Check sheet for the modelled part. Datum: model origin and axes. Units: mm. Face numbers are marked on the shaded views. A direction names the side the tool comes from. Coordinates: 2 decimals unless noted, no trailing zeros. Loops run counter-clockwise (first coordinate to the right, second up) from the corner with the lowest first, then second, coordinate; pieces in that order, holes last. Notation, with made-up numbers: (50.5, 59.25) -> (86.5, 59.25) arc R20 ccw to (86.5, 76.25) -> close; hole circle Ø3 at (82, -35.5). An arc over 180 degrees is marked (long way). Use one line per item in the form item = value.
from build123d import *

# Parameters (mm, degrees)
SKETCH1_R                       = 19.8
BOSS_EXTRUDE1_DEPTH             = 92
M4X0_7_TAPPED_HOLE1_D           = 3.3
M4X0_7_TAPPED_HOLE1_DEPTH       = 4
M4X0_7_TAPPED_HOLE1_CSINK_D     = 4.05
M4X0_7_TAPPED_HOLE1_CSINK_ANGLE = 90
M4X0_7_TAPPED_HOLE1_TIP         = 0.991420021
SKETCH6_R                       = 4
BOSS_EXTRUDE2_DEPTH             = 24
CHAMFER1_SIZE                   = 3
SKETCH7_W                       = 3.175
SKETCH7_H                       = 3.175
CUT_EXTRUDE1_DEPTH              = 19
CUT_EXTRUDE2_START              = -0.9
SKETCH8_R                       = 4
SKETCH8_R_2                     = 3.8
CUT_EXTRUDE2_DEPTH              = 0.9


with BuildPart() as part:
    # Sketch1 → Boss-Extrude1 (new body)
    with BuildSketch(Plane.XY):
        Circle(SKETCH1_R)
    extrude(amount=BOSS_EXTRUDE1_DEPTH)

    # M4x0.7 Tapped Hole1
    with Locations(Plane(origin=(0, 0, 0), x_dir=(-1, 0, 0), z_dir=(0, 0, -1))):
        with Locations((0, 12.5), (-12.5, 0), (0, -12.5), (12.5, 0)):
            CounterSinkHole(M4X0_7_TAPPED_HOLE1_D / 2, M4X0_7_TAPPED_HOLE1_CSINK_D / 2, depth=M4X0_7_TAPPED_HOLE1_DEPTH, counter_sink_angle=M4X0_7_TAPPED_HOLE1_CSINK_ANGLE)
            with Locations((0, 0, -(M4X0_7_TAPPED_HOLE1_DEPTH + M4X0_7_TAPPED_HOLE1_TIP / 2))):  # 118° drill point
                Cone(0, M4X0_7_TAPPED_HOLE1_D / 2, M4X0_7_TAPPED_HOLE1_TIP, mode=Mode.SUBTRACT)

    # Sketch6 → Boss-Extrude2 (add)
    with BuildSketch(Plane(origin=(0, 0, 0), x_dir=(-1, 0, 0), z_dir=(0, 0, -1))):
        Circle(SKETCH6_R)
    extrude(amount=BOSS_EXTRUDE2_DEPTH)

    # Chamfer1
    chamfer1_edges = [part.edges().sort_by_distance(p)[0] for p in [
        (-19.8, 0, 0),
    ]]
    chamfer(chamfer1_edges, length=CHAMFER1_SIZE)

    # Sketch7 → Cut-Extrude1 (cut)
    with BuildSketch(Plane(origin=(0, 0, -24), x_dir=(-1, 0, 0), z_dir=(0, 0, -1))):
        with Locations((0, 4)):
            Rectangle(SKETCH7_W, SKETCH7_H)
    extrude(amount=-CUT_EXTRUDE1_DEPTH, mode=Mode.SUBTRACT)

    # Sketch8 → Cut-Extrude2 (cut)
    with BuildSketch(Plane(origin=(0, 0, -22), x_dir=(-1, 0, 0), z_dir=(0, 0, -1)).offset(CUT_EXTRUDE2_START)):
        with Locations(Location((0, 0, 0), (0, 0, 113.382964427))):
            Circle(SKETCH8_R)
        Circle(SKETCH8_R_2, mode=Mode.SUBTRACT)
    extrude(amount=CUT_EXTRUDE2_DEPTH, mode=Mode.SUBTRACT)


solid = part.part
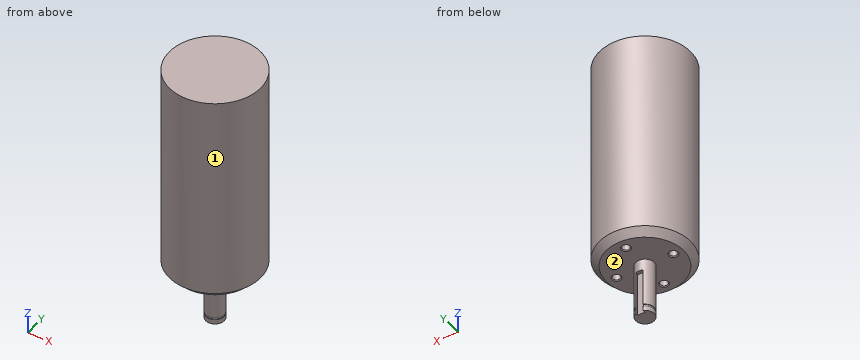
(1) Go/stop test with flat-tipped pins: P1, Ø0.8, axis at x = -0.5, y = 3.5, coming from the -Z side; P2, Ø10, axis at x = 7, y = 15.5, coming from the -Z side; P3, Ø1, axis at y = 3, z = -17.5, coming from the -X side; P4, Ø10, axis at x = -8, y = -1, coming from the -Z side. Record where each tip stops, or that it passes through.
Established:
P1 = -5
P2 = 0
P3 = -3.12
P4 = -24
(2) Section check A-A, the plane z = 10. Record the boundary of the cut face in (x, y), plus the area to 3 significant figures.
Established:
outline = circle Ø39.6 at (0, 0)
area = 1,230 mm²
(3) Scan lines: line 1 along Z through (x, y) = (-10.5, -4); line 2 along Y through (x, z) = (12.5, 1.5); line 3 along X through (y, z) = (0, 2.9). Record each from-to range of solid material in increasing order.
Established:
line_1 = 0 to 92
line_2 = -13.37 to -1.65, 1.65 to 13.37
line_3 = -19.7 to -14.15, -10.85 to 10.85, 14.15 to 19.7
(4) Tool access check on the marked faces 1 and 2. Record the directions out of +Z, -Z, +X, -X, +Y, -Y that give a thin tool (end or side, any length) a straight path to the whole face; none if there is none.
Established:
face_1 = +Z, -Z
face_2 = -Z
